Autodesk Inventor part; units mm, degrees
ref_plane "YZ Plane" through (0, 0, 0) normal (1, 0, 0) x (0, 1, 0)
ref_plane "XZ Plane" through (0, 0, 0) normal (0, 1, 0) x (-1, 0, 0)
ref_plane "XY Plane" through (0, 0, 0) normal (0, 0, 1) x (1, 0, 0)
ref_plane "Work Plane1" through (0, 0, 0) normal (0, 0, 1) x (1, 0, 0)
ref_plane "Work Plane2" through (0, 110, 380) normal (0, -1, 0) x (-1, 0, 0)
sketch "Sketch1" plane through (0, 0, 0) normal (0, 0, 1) x (1, 0, 0)
  line L0 (0, 0) -> (0, -840)
  line L1 (0, 0) -> (-100, 0)
  line L2 (-100, 0) -> (-100, -140)
  line L3 (-10, -140) -> (-100, -140)
  line L4 (-10, -140) -> (-10, -700)
  line L5 (-10, -700) -> (-100, -700)
  line L6 (-100, -700) -> (-100, -840)
  line L7 (0, -840) -> (-100, -840)
  line L8 (-100, -140) -> (-100, -700)
  line L9 (-100, -420) -> (0, -420)
extrude "Plate1" add sketch "Sketch1" against normal blind 1.5 contours L0 L9 L4 L3 L2 L1 | L9 L8 L3 L4
ref_plane "Work Plane3" through (0, 111.5, 380) normal (0, -1, 0) x (-1, 0, 0)
sketch "Sketch2" plane through (0, 111.5, 380) normal (0, -1, 0) x (-1, 0, 0)
  line L0 (0, 380) -> (100, 380)
  line L1 (100, 380) -> (100, -18.5)
  line L2 (100, -18.5) -> (0, -18.5)
  line L3 (0, -18.5) -> (0, 380)
edge flange "Flange1" height 400 angle 90 thickness 1.5 bend radius 110 thickness toward (0, -1, 0) relief tear relief width 1.5 relief depth 0.75 edges at (-50, 0, 0) wall of the first edge with corners at (0, 111.5, 0) (-100, 111.5, 0) (-100, 111.5, 398.5) (0, 111.5, 398.5)
bend "Bend1"
corner "Corner1"
equation "\"d0\" = Thickness"
equation "\"d2\" = BendReliefWidth"
equation "\"d3\" = BendReliefDepth"
equation "\"d4\" = MinimumRemnant"
equation "\"d5\" = TransitionRadius"
equation "\"d9\" = CornerReliefSize"
equation "\"d10\" = GapSize"
equation "\"d11\" = JacobiRadiusSize"
equation "\"BendRadius\" = Thickness"
equation "\"BendReliefWidth\" = Thickness"
equation "\"BendReliefDepth\" = 0.5 * Thickness"
equation "\"CornerReliefSize\" = 4 * Thickness"
equation "\"MinimumRemnant\" = 2 * Thickness"
equation "\"TransitionRadius\" = BendRadius"
equation "\"JacobiRadiusSize\" = BendRadius"
equation "\"GapSize\" = Thickness"
properties part number "CARCASA_ALUM_9"
For this review, take the finished solid that the model builds, in its own axes (mm). A direction names the side the tool comes from. Coordinates: 2 decimals unless noted, no trailing zeros. Order: outer loops, then holes, each group sorted by start corner. A loop starts at its lowest first (then second) coordinate and runs counter-clockwise, first axis right, second up. Notation, with made-up numbers: (-7.5, 18.5) - (29.5, 18.5) arc R27 ccw to (29.5, 48.5) - close; hole circle Ø1 at (-1, 42.25). An arc over 180 degrees is marked (long way). Answer as a JSON object with one key per item and string values. Group by question number.
1. Clearance check with flat-ended pins moving along their axes: P1, Ø6, axis at x = -13.5, z = 314, coming from the -Y side; P2, Ø1.5, axis at x = -56.5, y = 31, coming from the -Z side. State where each tip first meets the part, or that it passes through.
2. For faces 1 (the flat face through (-51, -207, -1.5)), 2 (the flat face through (-51, -207, 0)), list the 3-axis set-ups (+Z, -Z, +X, -X, +Y, -Y) from which the entire face can be reached by the end or side of a thin tool; tool diameter is ignored.
3. We need section B-B on z = 294.5. State the section outline as (x, y) points.
4. We need section A-A on x = -51.5. State the section outline as (y, z) points, then the cut area to 3 significant figures.
5. For probe 1 along Y at (x, z) = (-76, 225.5); probe 2 along Z at (x, y) = (-49, -281); probe 3 along Z at (x, y) = (-92, 55), list the stretches that pass through material, from the lowest coordinate up.
6. We need section C-C on y = -90.5. State the section outline as (x, z) points, then the cut area to 3 significant figures.
Final values:
{
 "1": {"P1": "y = 110", "P2": "z = 2.68"},
 "2": {"face 1": "-Z, +X, -X, +Y, -Y", "face 2": "+Z, +X, -X, -Y"},
 "3": {"outline": "(-100, 110) - (0, 110) - (0, 111.5) - (-100, 111.5) - close"},
 "4": {"outline": "(-420, -1.5) - (0, -1.5) arc R111.5 ccw to (111.5, 110) - (111.5, 398.5) - (110, 398.5) - (110, 110) arc R110 cw to (0, 0) - (-420, 0) - close", "area": "1,320 mm²"},
 "5": {"probe 1": "110 to 111.5", "probe 2": "-1.5 to 0", "probe 3": "13.01 to 14.74"},
 "6": {"outline": "(-100, -1.5) - (0, -1.5) - (0, 0) - (-100, 0) - close", "area": "150 mm²"}
}
